The figure shows three views and two pictorial views of one solid part (mm, origin at its lowest corner). Answer the questions. Coordinates: 2 decimals unless noted, no trailing zeros. Write each loop counter-clockwise with the first axis right and the second up, starting at its lowest first coordinate (ties: lowest second). Pieces come first, ordered by that corner, then holes. Notation, with made-up numbers: M -33.5,85 L 24.5,85 A15 cw 24.5,98 Z; hole C 33.5,76.5 d9. An arc over 180 degrees is marked long. Use a Markdown table: item, result. Add a question column.
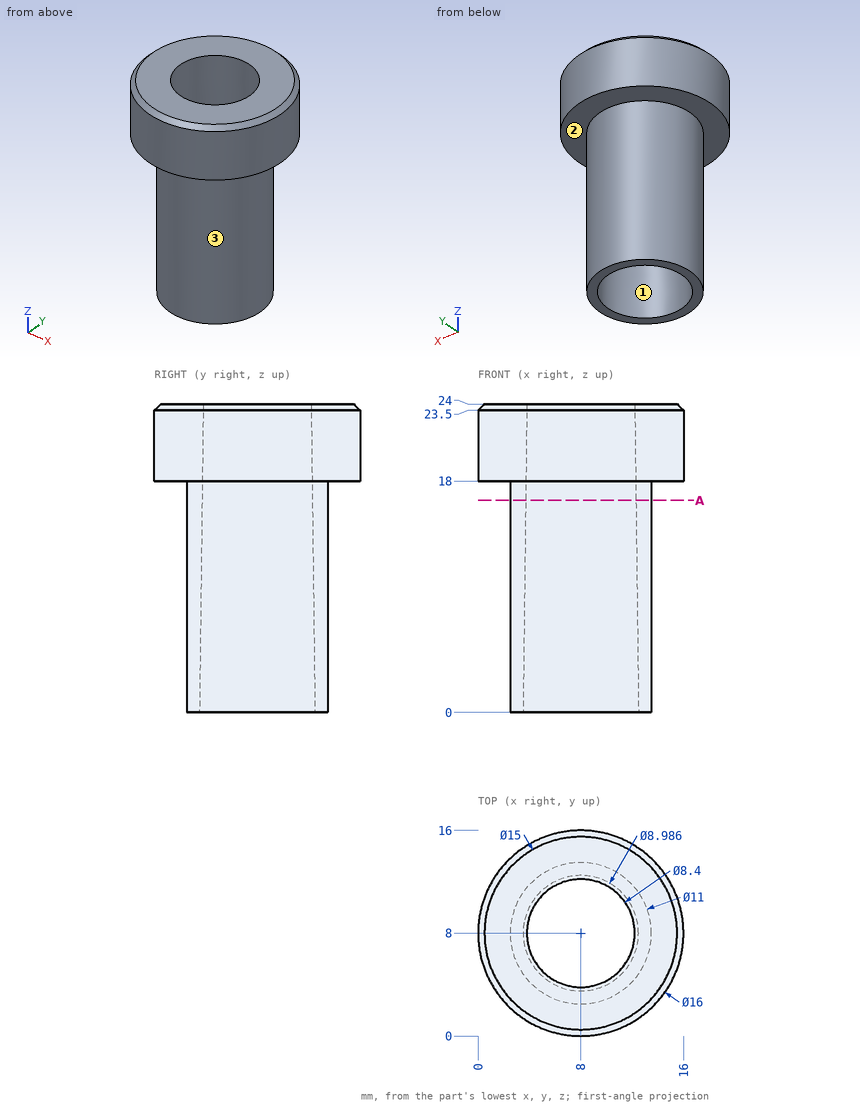
Item 1: Determine the mould class of the marked faces 1, 2 and 3 for opening direction X: pulls with the +X half, pulls with the -X half, needs draft (parallel to the pull), parting line crosses it, or undercut.
Item 2: Consider probe 1 along Z at (x, y) = (3, 4.75); probe 2 along X at (y, z) = (9, 13.25) (1 decimal); probe 3 along X at (y, z) = (9.5, 13.5). Determine where each line is inside the solid, lowest interval first.
Item 3: Find section A-A on z = 16.5. Give the vertices of the cut face in (x, y).
Item 4: Each of these flat-tipped pins is pushed along its axis until it touches: pin 1 (5 mm diameter, centred on x = 4.5, z = 3.5, fed in from -Y); pin 2 (1.5 mm diameter, centred on x = 7, z = 12.5, fed in from -Y); pin 3 (3 mm diameter, centred on y = 7, z = 5, fed in from -X). Where does it stop, or does it pass through?
Geometry says:
| question | item | result |
|---|---|---|
| 1 | face 1 | undercut |
| 1 | face 2 | needs draft |
| 1 | face 3 | parting line crosses it |
| 2 | probe 1 | z = 18 to 24 |
| 2 | probe 2 | x = 2.6 to 3.8, 12.2 to 13.4 |
| 2 | probe 3 | x = 2.71 to 3.94, 12.06 to 13.29 |
| 3 | outline | C 8,8 d11; hole C 8,8 d8.58 |
| 4 | pin 1 | stops at y = 2.59 |
| 4 | pin 2 | stops at y = 2.51 |
| 4 | pin 3 | stops at x = 2.5 |
